```python
from build123d import *

# Parameters (mm, degrees)
BOSS_EXTRUDE1_DEPTH     = 10
SKETCH2_R               = 1.5
CUT_EXTRUDE1_DEPTH      = 1
CUT_EXTRUDE1_DEPTH_BACK = 121
BOSS_EXTRUDE2_START     = -20
SKETCH5_W               = 6
SKETCH5_H               = 12
SKETCH5_R               = 1.25
BOSS_EXTRUDE2_DEPTH     = 10
LPATTERN1_COUNT         = 2
LPATTERN1_PITCH         = 40
LPATTERN1_COUNT_DIR2    = 2
LPATTERN1_PITCH_DIR2    = 40
BOSS_EXTRUDE4_DEPTH     = 18
CHAMFER1_SIZE           = 15


with BuildPart() as part:
    # Sketch1 → Boss-Extrude1 (new body)
    with BuildSketch(Plane(origin=(0, 0, 0), x_dir=(1, 0, 0), z_dir=(0, 1, 0))):
        with BuildLine():
            Line((-60, 0), (-60, 60))
            Line((-60, 60), (60, 60))
            Line((60, 60), (60, 0))
            ThreePointArc((60, 0), (0, -60), (-60, 0))
        make_face()
    extrude(amount=BOSS_EXTRUDE1_DEPTH)

    # Sketch2 → Cut-Extrude1 (cut, two sides)
    with BuildSketch(Plane.ZY.offset(60)) as cut_extrude1_sk:
        with Locations((-55, 5)):
            Circle(SKETCH2_R)
    extrude(amount=CUT_EXTRUDE1_DEPTH, mode=Mode.SUBTRACT)
    extrude(cut_extrude1_sk.sketch, amount=-CUT_EXTRUDE1_DEPTH_BACK, mode=Mode.SUBTRACT)

    # Sketch5 → Boss-Extrude2 (add)
    with BuildSketch(Plane.ZY.offset(60).offset(BOSS_EXTRUDE2_START)):
        with Locations((-44.29, 16)):
            Rectangle(SKETCH5_W, SKETCH5_H)
        with Locations((-44.29, 16)):
            Circle(SKETCH5_R, mode=Mode.SUBTRACT)
        with Locations((-15.71, 16)):
            Rectangle(SKETCH5_W, SKETCH5_H)
        with Locations((-15.71, 16)):
            Circle(SKETCH5_R, mode=Mode.SUBTRACT)
    boss_extrude2 = extrude(amount=-BOSS_EXTRUDE2_DEPTH)

    # LPattern1: Boss-Extrude2 2 × 2
    with Locations(*[(i * LPATTERN1_PITCH, 0, j * LPATTERN1_PITCH_DIR2) for i in range(LPATTERN1_COUNT) for j in range(LPATTERN1_COUNT_DIR2) if (i, j) != (0, 0)]):
        add(boss_extrude2)

    # Sketch9 → Boss-Extrude4 (add)
    with BuildSketch(Plane.XZ):
        Polygon((-53.548293043, -27.012784213), (-43.443719976, -21.178906233), (-41.83944897, -23.957585125), (-51.944022036, -29.791463105), align=None)
        Polygon((-9.957561883, -1.845663844), (0.147011183, 3.988214136), (1.75128219, 1.209535244), (-8.353290877, -4.624342736), align=None)
    extrude(amount=BOSS_EXTRUDE4_DEPTH)

    # Chamfer1
    chamfer1_edges = [part.edges().sort_by_distance(p)[0] for p in [
        (-46.891735503, 0, -26.874524115),
        (-3.301004344, 0, -1.707403746),
    ]]
    chamfer(chamfer1_edges, length=CHAMFER1_SIZE)


solid = part.part
```
The model under review builds one solid part; all positions refer to its coordinate system, in mm. A direction names the side the tool comes from. Coordinates: 2 decimals unless noted, no trailing zeros. Write each loop counter-clockwise with the first axis right and the second up, starting at its lowest first coordinate (ties: lowest second). Pieces come first, ordered by that corner, then holes. Notation, with made-up numbers: (57.5, -0.75) - (102.5, -0.75) arc R11 cw to (102.5, 8.25) - close; hole circle Ø11 at (30.25, -17). An arc over 180 degrees is marked (long way). Answer in a Markdown table with one row per item. Add a question column.
Q1. For faces 4 (the face through (3.62, -6.87, -2.03)), 5 (the face through (5, 16, -1.29)), 6 (the face through (0, 16, -6)), 7 (the face through (-3.23, -16.479, -1.667)), 8 (the face through (-40, 16, -46)), list the 3-axis set-ups (+Z, -Z, +X, -X, +Y, -Y) from which the entire face can be reached by the end or side of a thin tool; tool diameter is ignored.
Q2. Consider section D-D on x = 47. Give the boundary of the cut face in (y, z), then the cut area to 3 significant figures.
Q3. Draft analysis for pull direction Y (two halves, no side actions). For faces 1 (the face through (-35, 16, -12.71)), 2 (the face through (-35, 22, -4)), 3 (the face through (-48, -18, -26)), state which applies: +Y half, -Y half, draft (parallel to the pull), parting line (faces both ways), or undercut.
Q4. Consider section C-C on y = -13.5. Give the boundary of the cut face in (x, z), then the cut area to 3 significant figures.
Q5. To check wall thickness, follow line 1 along Z through (x, y) = (-36.5, 11); line 2 along Y through (x, z) = (-34, -4); line 3 along Y through (x, z) = (4.5, -38). State the ranges of each line that lie inside material, in increasing order. Write a range as from..to.
Q6. Consider section B-B on y = 19.5. Give the number of separate pieces and of enclosed holes in the cut face, then the cut area to 3 significant figures.
Q7. Clearance check with flat-ended pins moving along their axes: pin 1 (11 mm diameter, centred on x = -37.5, y = 16, fed in from -Z); pin 2 (5 mm diameter, centred on x = -33.5, y = 15.5, fed in from +Z); pin 3 (8 mm diameter, centred on x = -19.5, z = -2.5, fed in from +Y). State where each tip first meets the part, or that it passes through.
Q8. Consider section A-A on y = 5. Give the boundary of the cut face in (x, z).
Answers below:
| question | item | result |
|---|---|---|
| 1 | face 4 | +Z, +X, -Y |
| 1 | face 5 | +X, -X, +Y |
| 1 | face 6 | +Z, -Z, +Y |
| 1 | face 7 | -Z, +X, -Y |
| 1 | face 8 | +Z, -Z, -X, +Y |
| 2 | outline | (0, -60) - (10, -60) - (10, 37.3) - (0, 37.3) - close; hole circle Ø3 at (5, -55) |
| 2 | area | 966 mm² |
| 3 | face 1 | draft |
| 3 | face 2 | +Y half |
| 3 | face 3 | -Y half |
| 4 | outline | (-53.55, -27.01) - (-51.19, -31.09) - (-41.09, -25.26) - (-43.44, -21.18) - close; (-9.96, -1.85) - (-7.6, -5.92) - (2.5, -0.09) - (0.15, 3.99) - close |
| 4 | area | 110 mm² |
| 5 | line 1 | -47.29..-41.29, -18.71..-12.71, -7.29..-1.29, 21.29..27.29 |
| 5 | line 2 | 0..14.78, 17.22..22 |
| 5 | line 3 | 0..10 |
| 6 | separate pieces | 8 |
| 6 | enclosed holes | 0 |
| 6 | area | 480 mm² |
| 7 | pin 1 | z = -47.29 |
| 7 | pin 2 | z = 27.29 |
| 7 | pin 3 | y = 10 |
| 8 | outline | (-60, -60) - (60, -60) - (60, -56.5) - (-60, -56.5) - close; (-60, -53.5) - (60, -53.5) - (60, 0) arc R60 ccw to (-60, 0) - close |
